from build123d import *

# Parameters (mm, degrees)
F0_W     = 100
F0_H     = 100
F0_R     = 2
F1_DEPTH = 10
F2_R     = 2
F3_DEPTH = 7
F4_R     = 10
F4_R_2   = 7.5
F5_DEPTH = 4
F4_R_3   = 5
F6_DEPTH = 7
F7_DEPTH = 25


with BuildPart() as f1:
    # F0 (on Top) → F1 (new body)
    with BuildSketch(Plane.XY):
        Rectangle(F0_W, F0_H)
        with Locations((-42.426407, -42.426407)):
            Circle(F0_R, mode=Mode.SUBTRACT)
        with Locations((42.426407, -42.426407)):
            Circle(F0_R, mode=Mode.SUBTRACT)
        with Locations((-42.426407, 42.426407)):
            Circle(F0_R, mode=Mode.SUBTRACT)
        with Locations((42.426407, 42.426407)):
            Circle(F0_R, mode=Mode.SUBTRACT)
    extrude(amount=F1_DEPTH)

    # F2 (on face) → F3 (join)
    with BuildSketch(Plane.XY.offset(10)):
        with Locations((14.142136, -14.142136)):
            Circle(F2_R)
        with Locations((21.213203, -21.213203)):
            Circle(F2_R)
        with Locations((28.284271, -28.284271)):
            Circle(F2_R)
        with Locations((35.355339, -35.355339)):
            Circle(F2_R)
        with Locations((14.142136, 14.142136)):
            Circle(F2_R)
        with Locations((21.213203, 21.213203)):
            Circle(F2_R)
        with Locations((28.284271, 28.284271)):
            Circle(F2_R)
        with Locations((35.355339, 35.355339)):
            Circle(F2_R)
        with Locations((-14.142136, 14.142136)):
            Circle(F2_R)
        with Locations((-21.213203, 21.213203)):
            Circle(F2_R)
        with Locations((-28.284271, 28.284271)):
            Circle(F2_R)
        with Locations((-35.355339, 35.355339)):
            Circle(F2_R)
        with Locations((-14.142136, -14.142136)):
            Circle(F2_R)
        with Locations((-21.213203, -21.213203)):
            Circle(F2_R)
        with Locations((-28.284271, -28.284271)):
            Circle(F2_R)
        with Locations((-35.355339, -35.355339)):
            Circle(F2_R)
    extrude(amount=F3_DEPTH)

    # F4 (on face) → F5 (join)
    with BuildSketch(Plane.XY.offset(10)):
        Circle(F4_R)
        Circle(F4_R_2, mode=Mode.SUBTRACT)
    extrude(amount=F5_DEPTH)

    # F4 (on face) → F6 (join)
    with BuildSketch(Plane.XY.offset(10)):
        Circle(F4_R_2)
        Circle(F4_R_3, mode=Mode.SUBTRACT)
    extrude(amount=F6_DEPTH)

    # F4 (on face) → F7 (cut)
    with BuildSketch(Plane.XY.offset(10)):
        Circle(F4_R_3)
    extrude(amount=-F7_DEPTH, mode=Mode.SUBTRACT)


solid = f1.part
Work out the finished part from the listing and answer in its coordinate system (mm). A direction names the side the tool comes from. Give positions to 0.01 mm unless a question says otherwise; leave off trailing zeros. Order: outer loops, then holes, each group sorted by start corner. A loop starts at its lowest first (then second) coordinate and runs counter-clockwise, first axis right, second up. Notation, with made-up numbers: (57.25, -27.5) -> (78.25, -27.5) arc R8 cw to (78.25, -23.5) -> close; hole circle Ø2 at (-22, 86.5). An arc over 180 degrees is marked (long way). Answer as a JSON object with one key per item and string values. Group by question number.
1. The mould has two halves that part along Y. Classify faces 3 (the flat face through (35, 35, 17)), 4 (the cylindrical face through (-7.493, 0.33, 15.479)), 5 (the cylindrical face through (-12.295, 13.376, 13.451)): released by +Y, released by -Y, zero draft, split by the parting line, or undercut.
2. Consider line 1 along Y through (x, z) = (-43, 8); line 2 along X through (y, z) = (28, 15.25); line 3 along Y through (x, z) = (-14, 11.25). Determine where each line is inside the solid, lowest interval first. Write a range as [from, to].
3. Flat-ended cylindrical pins translate along their axes: pin 1 Ø9 at (x, y) = (0, 0) entering from +Z; pin 2 Ø4 at (x, z) = (13.5, 13) entering from -Y; pin 3 Ø10 at (x, y) = (2, 2) entering from +Z. Find the tip coordinate at first contact, or state that the pin passes through.
4. Section C-C on z = 12.25 is taken. Count the separate pieces of the cut face and the enclosed holes in it, plus the area to 3 significant figures.
5. Section A-A on y = 0 is taken. Determine the outline of the cut face in (x, z), plus the area to 3 significant figures.
6. A tool of negligible diameter and unlimited length cuts with its end or side. For faces 1 (the cylindrical face through (29.21, 26.51, 13.45)), 2 (the flat face through (-14, -14, 17)), from which of +Z, -Z, +X, -X, +Y, -Y can it reach the whole face along a straight path? Write none if from no direction.
Result sheet:
{
 "1": {"face 3": "zero draft", "face 4": "split by the parting line", "face 5": "undercut"},
 "2": {"line 1": "y = [-50, -44.34], [-40.51, 40.51], [44.34, 50]", "line 2": "x = [-30.26, -26.3], [26.3, 30.26]", "line 3": "y = [-16.14, -12.15], [12.15, 16.14]"},
 "3": {"pin 1": "passes through", "pin 2": "stops at y = -16.14", "pin 3": "stops at z = 17"},
 "4": {"separate pieces": "17", "enclosed holes": "1", "area": "437 mm^2"},
 "5": {"outline": "(-50, 0) -> (-5, 0) -> (-5, 17) -> (-7.5, 17) -> (-7.5, 14) -> (-10, 14) -> (-10, 10) -> (-50, 10) -> close; (5, 0) -> (50, 0) -> (50, 10) -> (10, 10) -> (10, 14) -> (7.5, 14) -> (7.5, 17) -> (5, 17) -> close", "area": "955 mm^2"},
 "6": {"face 1": "+Z", "face 2": "+Z, +X, -X, +Y, -Y"}
}
